Geometry: see drawing. Coordinates: mm, zero at the bounding-box minimum. Round coordinates to 2 decimals unless told otherwise and drop trailing zeros. Write each loop counter-clockwise with the first axis right and the second up, starting at its lowest first coordinate (ties: lowest second). Pieces come first, ordered by that corner, then holes.
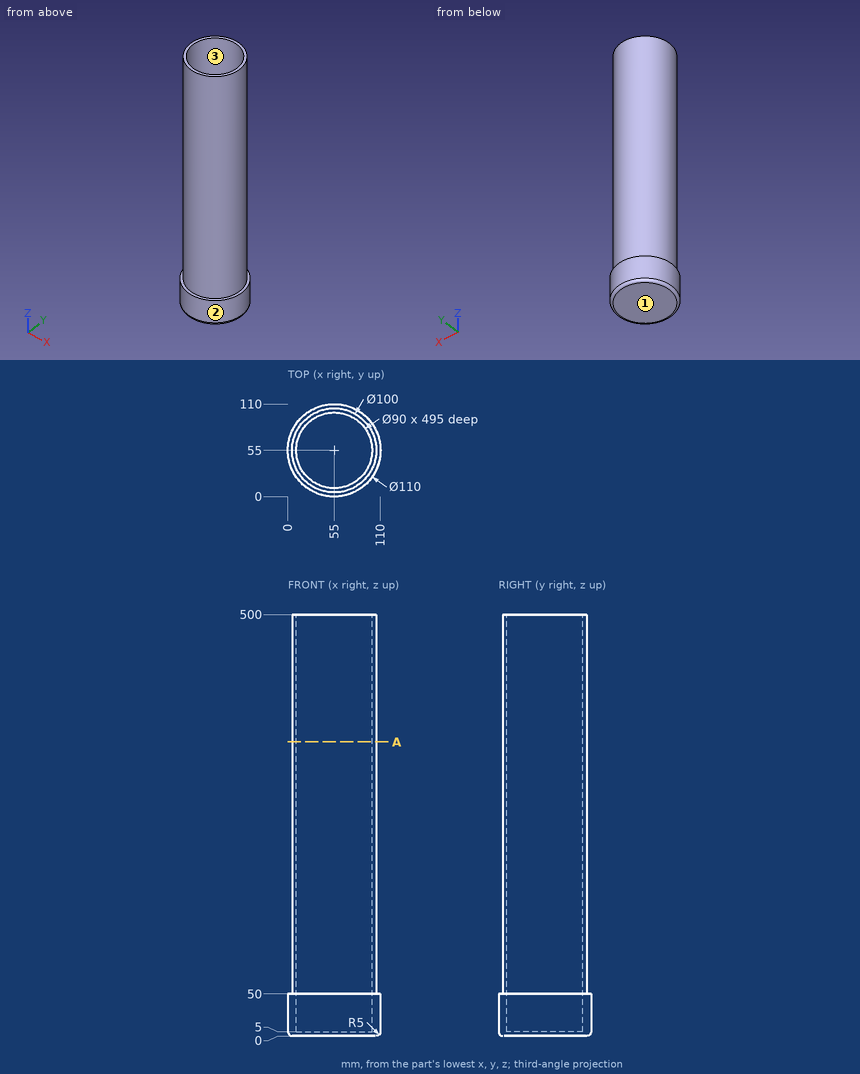
1) Material intervals for line 1 (Y direction, x = 55, z = 216.5); line 2 (Z direction, x = 14, y = 60.5), sorted ascending.
Taken from the geometry:
line 1: y = 5 to 10, 100 to 105
line 2: z = 0 to 5
2) Section query A-A on z = 349. Return the cut outline in (x, y).
Taken from the geometry:
outline: circle Ø100 at (55, 55); hole circle Ø90 at (55, 55)
3) Contact query for flat-ended pins moving along their axis: P1, Ø6, axis at x = 25, z = 144, coming from the -Y side; P2, Ø5, axis at x = 84, y = 24.5, coming from the +Z side; P3, Ø8, axis at x = 38, z = 156.5, coming from the +Y side. Output: stop coordinate, or through.
Taken from the geometry:
P1: stops at y = 12.92
P2: stops at z = 5
P3: stops at y = 103.28
4) Pull-direction query (X, two-part tool) for the marked faces 1, 2 and 3; classes: released by +X, released by -X, zero draft, split by the parting line, or undercut.
Taken from the geometry:
face 1: zero draft
face 2: split by the parting line
face 3: undercut
